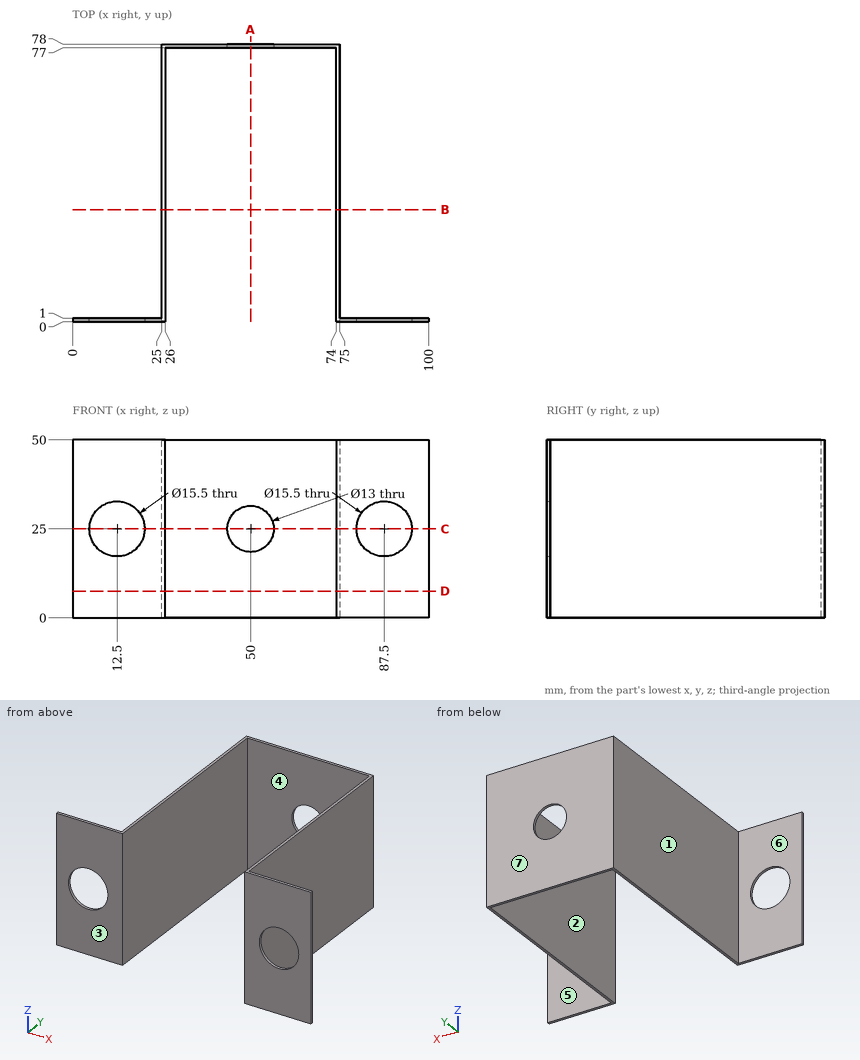
Geometry check sheet. Reference: drawing and pictorial views, mm from the part's lowest x, y, z. A direction names the side the tool comes from. Round coordinates to 2 decimals unless told otherwise and drop trailing zeros. Order: outer loops, then holes, each group sorted by start corner. A loop starts at its lowest first (then second) coordinate and runs counter-clockwise, first axis right, second up. Notation, with made-up numbers: (-20.75, 29.25) - (0.25, 29.25) arc R16 cw to (0.25, 55.25) - close; hole circle Ø6 at (59, -29.5). An arc over 180 degrees is marked (long way). Use a Markdown table: item, result. Add a question column.
1) Set-up check for the marked faces 4, 5, 6 and 7: record each of +Z, -Z, +X, -X, +Y, -Y from which the full face is reachable in a straight line by a thin tool's end or side.
2) Gauge pin test, flat ends, axial feed: P1, Ø20, axis at x = 12.5, z = 25, coming from the +Y side; P2, Ø5, axis at y = 69.5, z = 18, coming from the +X side; P3, Ø1.5, axis at y = 58, z = 33.5, coming from the -X side. Record the tip position at first contact, or that the pin passes through.
3) Section check A-A (x = 50). Record the cut outline in (y, z), then the cut area to 3 significant figures.
4) Thickness scan on line 1 along X through (y, z) = (0.2, 25); line 2 along X through (y, z) = (21.5, 45.5); line 3 along Z through (x, y) = (87.5, 0.3). Record the ranges inside material, lowest first.
5) Section check D-D (z = 7.5). Record the cut outline in (x, y), then the cut area to 3 significant figures.
6) Section check C-C (z = 25). Record the cut outline in (x, y).
7) Mould release check, pull along X, two halves, no side actions. Record for the marked faces 1, 2 and 3: released by +X, released by -X, zero draft, split by the parting line, or undercut.
8) Section check B-B (y = 31.5). Record the cut outline in (x, z).
Established:
| question | item | result |
|---|---|---|
| 1 | face 4 | +Z, -Z, -Y |
| 1 | face 5 | +Z, -Z, +X, +Y |
| 1 | face 6 | +Z, -Z, -X, +Y |
| 1 | face 7 | +Z, -Z, +X, -X, +Y |
| 2 | P1 | y = 1 |
| 2 | P2 | x = 75 |
| 2 | P3 | x = 25 |
| 3 | outline | (77, 0) - (78, 0) - (78, 18.5) - (77, 18.5) - close; (77, 31.5) - (78, 31.5) - (78, 50) - (77, 50) - close |
| 3 | area | 37.0 mm2 |
| 4 | line 1 | 0 to 4.75, 20.25 to 26, 74 to 79.75, 95.25 to 100 |
| 4 | line 2 | 25 to 26, 74 to 75 |
| 4 | line 3 | 0 to 17.25, 32.75 to 50 |
| 5 | outline | (0, 0) - (26, 0) - (26, 77) - (74, 77) - (74, 0) - (100, 0) - (100, 1) - (75, 1) - (75, 78) - (25, 78) - (25, 1) - (0, 1) - close |
| 5 | area | 254 mm2 |
| 6 | outline | (0, 0) - (4.75, 0) - (4.75, 1) - (0, 1) - close; (20.25, 0) - (26, 0) - (26, 77) - (43.5, 77) - (43.5, 78) - (25, 78) - (25, 1) - (20.25, 1) - close; (56.5, 77) - (74, 77) - (74, 0) - (79.75, 0) - (79.75, 1) - (75, 1) - (75, 78) - (56.5, 78) - close; (95.25, 0) - (100, 0) - (100, 1) - (95.25, 1) - close |
| 7 | face 1 | released by -X |
| 7 | face 2 | undercut |
| 7 | face 3 | zero draft |
| 8 | outline | (25, 0) - (26, 0) - (26, 50) - (25, 50) - close; (74, 0) - (75, 0) - (75, 50) - (74, 50) - close |
